Input: dimensioned drawing with shaded views. Units: mm. Origin: part minimum x, y, z. A direction names the side the tool comes from. Coordinates: 2 decimals unless noted, no trailing zeros. Loops run counter-clockwise (first coordinate to the right, second up) from the corner with the lowest first, then second, coordinate; pieces in that order, holes last.
Item 1: Section query D-D, the plane x = 26. Return the cut outline in (y, z) (1 decimal).
Item 2: Section query A-A, the plane y = 19.05. Return the cut outline in (x, z) (1 decimal).
Item 3: Reachability of the marked faces 1 and 2 from +Z, -Z, +X, -X, +Y, -Y: full face, straight path, thin tool, end or side. Return the list, or none.
Item 4: Pull-direction query (X, two-part tool) for the marked faces 3, 4, 5 and 6; classes: +X half, -X half, draft (parallel to the pull), parting line (faces both ways), or undercut.
Item 5: Section query B-B, the plane x = 19.05. Return the cut outline in (y, z) (1 decimal).
Item 6: Line query: probe 1 along Y at (x, z) = (19.05, 35.8); probe 2 along X at (y, z) = (13.75, 21.5) (1 decimal); probe 3 along Z at (x, y) = (18, 14.75) (1 decimal). Output: solid intervals per line, ascending.
Item 7: Pin query (flat end, axial travel): pin 1 Ø10 at (x, y) = (21.5, 15.5) entering from -Z (1 decimal); pin 2 Ø3 at (x, y) = (19.05, 19.05) entering from +Z. Return the tip coordinate at first contact, or that it passes through.
Item 8: Section query C-C, the plane z = 31. Return the cut outline in (x, y) (1 decimal), then the cut area to 3 significant figures.
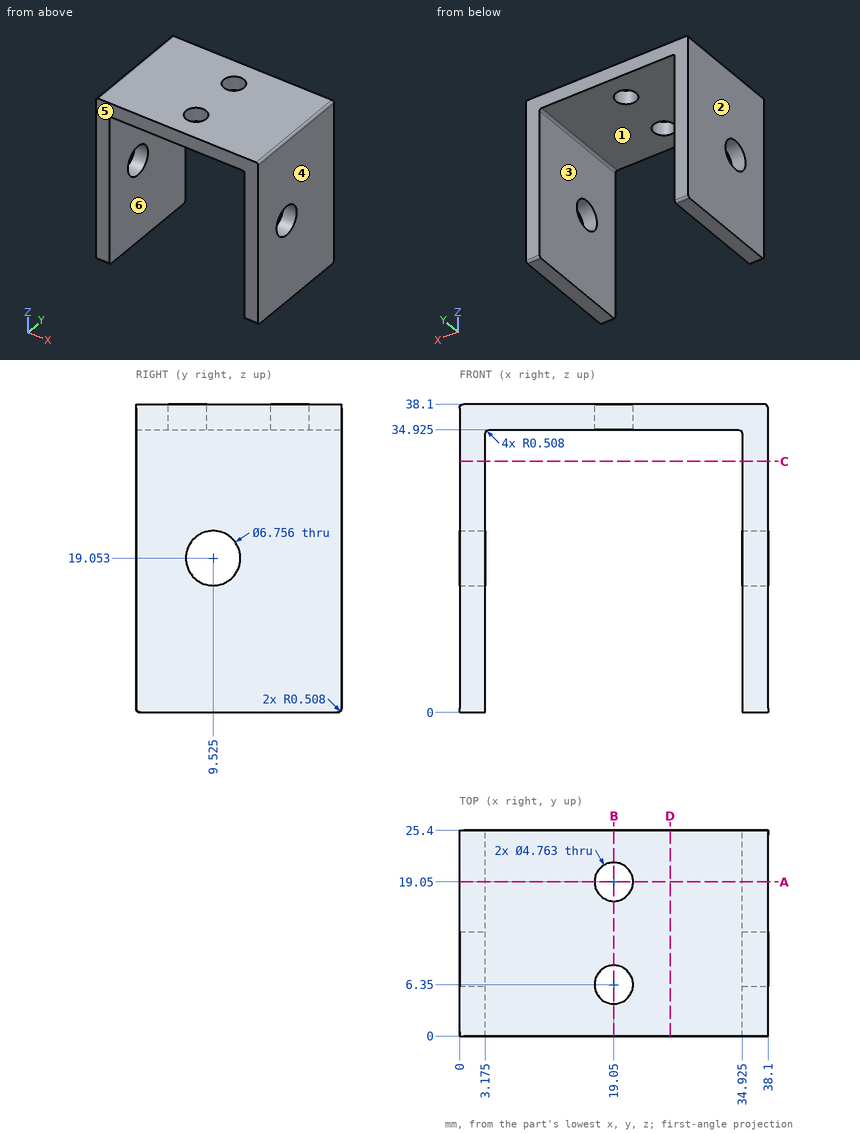
Verdict:
1. outline: (0, 34.9) - (25.4, 34.9) - (25.4, 38.1) - (0, 38.1) - close
2. outline: (0, 0) - (3.2, 0) - (3.2, 34.4) arc R0.5 cw to (3.7, 34.9) - (16.7, 34.9) - (16.7, 38.1) - (0.5, 38.1) arc R0.5 ccw to (0, 37.6) - close; (21.4, 34.9) - (34.4, 34.9) arc R0.5 cw to (34.9, 34.4) - (34.9, 0) - (38.1, 0) - (38.1, 37.6) arc R0.5 ccw to (37.6, 38.1) - (21.4, 38.1) - close
3. face 1: -Z, +Y, -Y
3. face 2: +Z, -Z, -X, +Y, -Y
4. face 3: undercut
4. face 4: +X half
4. face 5: draft
4. face 6: undercut
5. outline: (0, 34.9) - (4, 34.9) - (4, 38.1) - (0, 38.1) - close; (8.7, 34.9) - (16.7, 34.9) - (16.7, 38.1) - (8.7, 38.1) - close; (21.4, 34.9) - (25.4, 34.9) - (25.4, 38.1) - (21.4, 38.1) - close
6. probe 1: y = 0 to 3.97, 8.73 to 16.67, 21.43 to 25.4
6. probe 2: x = 0 to 3.2, 34.9 to 38.1
6. probe 3: z = 34.9 to 38.1
7. pin 1: stops at z = 34.9
7. pin 2: passes through
8. outline: (0, 0) - (3.2, 0) - (3.2, 25.4) - (0, 25.4) - close; (34.9, 0) - (38.1, 0) - (38.1, 25.4) - (34.9, 25.4) - close
8. area: 161 mm2
